```python
from build123d import *

# Parameters (mm, degrees)
SKETCH1_W           = 44
SKETCH1_H           = 23
BOSS_EXTRUDE1_DEPTH = 2
SKETCH2_W           = 20.7
SKETCH2_H           = 2
SKETCH2_W_2         = 30
SKETCH2_H_2         = 12.3
CUT_EXTRUDE1_DEPTH  = 2
SKETCH3_W           = 8
SKETCH3_H           = 2
BOSS_EXTRUDE2_DEPTH = 6


with BuildPart() as part:
    # Sketch1 → Boss-Extrude1 (new body)
    with BuildSketch(Plane(origin=(0, 0, 0), x_dir=(1, 0, 0), z_dir=(0, 1, 0))):
        Rectangle(SKETCH1_W, SKETCH1_H)
    extrude(amount=BOSS_EXTRUDE1_DEPTH)

    # Sketch2 → Cut-Extrude1 (cut)
    with BuildSketch(Plane(origin=(0, 2, 0), x_dir=(1, 0, 0), z_dir=(0, 1, 0))):
        with Locations((-1.65, 6.7)):
            Rectangle(SKETCH2_W, SKETCH2_H)
        with Locations((0, -3.35)):
            Rectangle(SKETCH2_W_2, SKETCH2_H_2)
    extrude(amount=-CUT_EXTRUDE1_DEPTH, mode=Mode.SUBTRACT)

    # Sketch3 → Boss-Extrude2 (add)
    with BuildSketch(Plane(origin=(0, 2, 0), x_dir=(1, 0, 0), z_dir=(0, 1, 0))):
        with Locations((-11, -10.5)):
            Rectangle(SKETCH3_W, SKETCH3_H)
        with Locations((0, -10.5)):
            Rectangle(SKETCH3_W, SKETCH3_H)
        with Locations((11, -10.5)):
            Rectangle(SKETCH3_W, SKETCH3_H)
    extrude(amount=BOSS_EXTRUDE2_DEPTH)


solid = part.part
```
Geometry: final body of the model. Coordinates: model frame, mm. A direction names the side the tool comes from. Coordinates: 2 decimals unless noted, no trailing zeros. Loops run counter-clockwise (first coordinate to the right, second up) from the corner with the lowest first, then second, coordinate; pieces in that order, holes last. Notation, with made-up numbers: (18.5, 76) -> (72.5, 76) arc R30 ccw to (72.5, 101) -> close; hole circle Ø10 at (1, 20). An arc over 180 degrees is marked (long way). Use a Markdown table: item, result. Add a question column.
(1) Section query C-C, the plane z = 8. Return loops of the section in (x, y), plus the area to 3 significant figures.
(2) Access query for faces 5 (the flat face through (-4, 5, 11)), 6 (the flat face through (-2, 1, -7.7)), 7 (the flat face through (-11, 8, 10)). Directions: +Z, -Z, +X, -X, +Y, -Y. A direction counts if a zero-diameter tool reaches every point of the face in a straight line with its end or side. Return the directions, or none.
(3) Mould query, pull axis X, two halves, no side actions, for faces 1 (the flat face through (-22, 1, 0)), 2 (the flat face through (22, 1, 0)), 3 (the flat face through (-12, 1, -7)), 4 (the flat face through (0, 2, -5)). Classes: pulls with the +X half, pulls with the -X half, needs draft (parallel to the pull), parting line crosses it, or undercut.
(4) Section query B-B, the plane x = 14.5. Return loops of the section in (y, z).
(5) Pin query (flat end, axial travel): pin 1 Ø1 at (y, z) = (5.5, 10) entering from +X; pin 2 Ø2 at (y, z) = (5.5, 11) entering from -X; pin 3 Ø1.6 at (x, z) = (5, 10.5) entering from +Y. Return the tip coordinate at first contact, or that it passes through.
(6) Section query D-D, the plane x = -1.5. Return loops of the section in (y, z).
(7) Line query: line 1 along Z through (x, y) = (8.5, 0.75); line 2 along X through (y, z) = (1.75, 3.75); line 3 along X through (y, z) = (0.5, -6.75). Output: solid intervals per line, ascending.
(8) Section query A-A, the plane y = 3. Return loops of the section in (x, z).
Answer:
| question | item | result |
|---|---|---|
| 1 | outline | (-22, 0) -> (-15, 0) -> (-15, 2) -> (-22, 2) -> close; (15, 0) -> (22, 0) -> (22, 2) -> (15, 2) -> close |
| 1 | area | 28.0 mm^2 |
| 2 | face 5 | +Z, -Z, +Y |
| 2 | face 6 | +Y, -Y |
| 2 | face 7 | +Z, -Z, +X, -X, +Y |
| 3 | face 1 | pulls with the -X half |
| 3 | face 2 | pulls with the +X half |
| 3 | face 3 | undercut |
| 3 | face 4 | needs draft |
| 4 | outline | (0, -11.5) -> (2, -11.5) -> (2, -2.8) -> (0, -2.8) -> close; (0, 9.5) -> (8, 9.5) -> (8, 11.5) -> (0, 11.5) -> close |
| 5 | pin 1 | stops at x = 15 |
| 5 | pin 2 | stops at x = -15 |
| 5 | pin 3 | stops at y = 2 |
| 6 | outline | (0, -11.5) -> (2, -11.5) -> (2, -7.7) -> (0, -7.7) -> close; (0, -5.7) -> (2, -5.7) -> (2, -2.8) -> (0, -2.8) -> close; (0, 9.5) -> (8, 9.5) -> (8, 11.5) -> (0, 11.5) -> close |
| 7 | line 1 | z = -11.5 to -7.7, -5.7 to -2.8, 9.5 to 11.5 |
| 7 | line 2 | x = -22 to -15, 15 to 22 |
| 7 | line 3 | x = -22 to -12, 8.7 to 22 |
| 8 | outline | (-15, 9.5) -> (-7, 9.5) -> (-7, 11.5) -> (-15, 11.5) -> close; (-4, 9.5) -> (4, 9.5) -> (4, 11.5) -> (-4, 11.5) -> close; (7, 9.5) -> (15, 9.5) -> (15, 11.5) -> (7, 11.5) -> close |
